from build123d import *

# Parameters (mm, degrees)
F0_R      = 2.125
F0_R_2    = 3.5
F0_R_3    = 13
F1_DEPTH  = 10
F2_W      = 30
F2_H      = 42.2
F2_R      = 3.5
F3_DEPTH  = 7
F4_R      = 3.5
F5_DEPTH  = 5
F6_R      = 6
F7_DEPTH  = 5
F8_W      = 30
F8_H      = 42.2
F8_R      = 3.5
F9_DEPTH  = 13
F10_R     = 2
F11_DEPTH = 42.201
F12_R     = 2


with BuildPart() as f1:
    # F0 (on Top) → F1 (new body)
    with BuildSketch(Plane.XY):
        Polygon((21.1, 21.1), (0, 21.1), (-21.1, 21.1), (-66.8, 21.1), (-66.8, 0), (-66.8, -21.1), (-21.1, -21.1), (0, -21.1), (21.1, -21.1), (21.1, 0), align=None)
        with Locations((-15.5, -15.5)):
            Circle(F0_R, mode=Mode.SUBTRACT)
        with Locations((15.5, -15.5)):
            Circle(F0_R, mode=Mode.SUBTRACT)
        with Locations((-51.8, 0)):
            Circle(F0_R_2, mode=Mode.SUBTRACT)
        Circle(F0_R_3, mode=Mode.SUBTRACT)
        with Locations((-15.5, 15.5)):
            Circle(F0_R, mode=Mode.SUBTRACT)
        with Locations((15.5, 15.5)):
            Circle(F0_R, mode=Mode.SUBTRACT)
    extrude(amount=F1_DEPTH)

    # F2 (on face) → F3 (join)
    with BuildSketch(Plane.XY.offset(10)):
        with Locations((-51.8, 0)):
            Rectangle(F2_W, F2_H)
        with Locations((-51.8, 0)):
            Circle(F2_R, mode=Mode.SUBTRACT)
    extrude(amount=F3_DEPTH)

    # F4 (on face) → F5 (cut)
    with BuildSketch(Plane.XY.offset(10)):
        with Locations((-15.5, 15.5)):
            Circle(F4_R)
        with Locations((15.5, 15.5)):
            Circle(F4_R)
        with Locations((15.5, -15.5)):
            Circle(F4_R)
        with Locations((-15.5, -15.5)):
            Circle(F4_R)
    extrude(amount=-F5_DEPTH, mode=Mode.SUBTRACT)

    # F6 (on face) → F7 (cut)
    with BuildSketch(Plane.XY.offset(17)):
        with Locations((-51.8, 0)):
            Circle(F6_R)
    extrude(amount=-F7_DEPTH, mode=Mode.SUBTRACT)

    # F8 (on face) → F9 (join)
    with BuildSketch(Plane(origin=(0, 0, 0), x_dir=(1, 0, 0), z_dir=(0, 0, -1))):
        with Locations((-51.8, 0)):
            Rectangle(F8_W, F8_H)
        with Locations((-51.8, 0)):
            Circle(F8_R, mode=Mode.SUBTRACT)
    extrude(amount=F9_DEPTH)

    # F10 (on face) → F11 (cut, through all)
    with BuildSketch(Plane.XZ.offset(21.1)):
        with Locations((-56.8, 2)):
            Circle(F10_R)
    extrude(amount=-F11_DEPTH, mode=Mode.SUBTRACT)

    # F12
    f12_edges = [f1.edges().sort_by_distance(p)[0] for p in [
        (21.1, 21.1, 5),
        (21.1, -21.1, 5),
        (-66.8, -21.1, 2),
        (-66.8, 21.1, 2),
    ]]
    fillet(f12_edges, radius=F12_R)


solid = f1.part
Build history of the part. All positions in model axes, mm. A direction names the side the tool comes from. Round coordinates to 2 decimals unless told otherwise and drop trailing zeros. Order: outer loops, then holes, each group sorted by start corner. A loop starts at its lowest first (then second) coordinate and runs counter-clockwise, first axis right, second up. Notation, with made-up numbers: M 35.25,3.5 L 45.25,3.5 A29 cw 45.25,35.5 Z; hole C -19,-23.75 d8. An arc over 180 degrees is marked long. Use CSV: the item, a comma, the result in double quotes. Start each with the question number.
(1) Cut at C-C on z = 2. List the corners of the cut face in (x, y) (3 decimals), then the cut area to 3 significant figures.
(2) Cut at B-B on x = -51.8. List the corners of the cut face in (y, z), then the cut area to 3 significant figures.
(3) Tool access for faces 4 (the face through (-36.8, 0, -6)), 5 (the face through (-66.23, 20.5, 1.79)), 6 (the face through (13.377, -15.407, 2.465)), 7 (the face through (-15, 0, 10)), 8 (the face through (-16, -18, 5)): list every direction of +Z, -Z, +X, -X, +Y, -Y with a clear straight run to the whole face (end or side of a thin tool).
(4) Drill centre lines: probe 1 along Y at (x, z) = (15.5, 2.35) (3 decimals); probe 2 along X at (y, z) = (-1, 5); probe 3 along X at (y, z) = (-15, 1). Where is each one in solid material? Low to high.
(5) Cut at D-D on x = -15.5. List the corners of the cut face in (y, z) (3 decimals), then the cut area to 4 significant figures.
(6) Cut at A-A on y = 15.5. List the corners of the cut face in (x, z) (3 decimals), then the cut area to 3 significant figures.
(7) Mould opens along Y. For faces 1 (the face through (-12.267, -16.841, 7.535)), 2 (the face through (-36.8, 0, 13)), 3 (the face through (-66.23, -20.5, 2.21)) say: +Y half, -Y half, draft (parallel to the pull), parting line (faces both ways), or undercut.
(8) Flat gauge pins, fed straight in: P1, Ø12, axis at y = 12, z = -1.5, coming from the +X side; P2, Ø2, axis at x = 15.5, y = 17, coming from the +Z side; P3, Ø6, axis at x = 10, y = -6, coming from the +Z side; P4, Ø7, axis at x = 15.5, y = -15.5, coming from the -Z side. Where does each tip first touch, or does it go through?
Findings:
1,outline,"M -66.8,-19.1 A2 ccw -64.8,-21.1 L -58.8,-21.1 L -58.8,21.1 L -64.8,21.1 A2 ccw -66.8,19.1 Z; M -54.8,-21.1 L 19.1,-21.1 A2 ccw 21.1,-19.1 L 21.1,19.1 A2 ccw 19.1,21.1 L -54.8,21.1 L -54.8,1.803 A3.5 cw long -54.8,-1.803 Z; hole C -15.5,-15.5 d4.25; hole C -15.5,15.5 d4.25; hole C 0,0 d26; hole C 15.5,-15.5 d4.25; hole C 15.5,15.5 d4.25"
1,area,"2,910 mm^2"
2,outline,"M -21.1,-13 L -3.5,-13 L -3.5,12 L -6,12 L -6,17 L -21.1,17 Z; M 3.5,-13 L 21.1,-13 L 21.1,17 L 6,17 L 6,12 L 3.5,12 Z"
2,area,"1,030 mm^2"
3,face 4,"-Z, +X, +Y, -Y"
3,face 5,"+Z, -Z, -X, +Y"
3,face 6,"+Z, -Z"
3,face 7,"+Z, +X, +Y, -Y"
3,face 8,"+Z"
4,probe 1,"y = -21.1 to -17.625, -13.375 to 13.375, 17.625 to 21.1"
4,probe 2,"x = -66.8 to -55.15, -48.45 to -12.96, 12.96 to 21.1"
4,probe 3,"x = -66.8 to -58.53, -55.07 to -17.57, -13.43 to 13.43, 17.57 to 21.1"
5,outline,"M -21.1,0 L -17.625,0 L -17.625,5 L -19,5 L -19,10 L -21.1,10 Z; M -13.375,0 L 13.375,0 L 13.375,5 L 12,5 L 12,10 L -12,10 L -12,5 L -13.375,5 Z; M 17.625,0 L 21.1,0 L 21.1,10 L 19,10 L 19,5 L 17.625,5 Z"
5,area,"309.5 mm^2"
6,outline,"M -66.8,-13 L -36.8,-13 L -36.8,0 L -17.625,0 L -17.625,5 L -19,5 L -19,10 L -36.8,10 L -36.8,17 L -66.8,17 Z; M -13.375,0 L 13.375,0 L 13.375,5 L 12,5 L 12,10 L -12,10 L -12,5 L -13.375,5 Z; M 17.625,0 L 21.1,0 L 21.1,10 L 19,10 L 19,5 L 17.625,5 Z; hole C -56.8,2 d4"
6,area,"1,350 mm^2"
7,face 1,"undercut"
7,face 2,"draft"
7,face 3,"-Y half"
8,P1,"stops at x = 21.1"
8,P2,"stops at z = 5"
8,P3,"stops at z = 10"
8,P4,"stops at z = 0"
